Could you check a few things on this model? Use its own coordinates, in mm. A direction names the side the tool comes from. Coordinates: 2 decimals unless noted, no trailing zeros. Loops run counter-clockwise (first coordinate to the right, second up) from the corner with the lowest first, then second, coordinate; pieces in that order, holes last.
1) Imagine slicing it at A-A on x = 0. Please give me the cut outline in (y, z).
2) Imagine slicing it at B-B on z = 0. Please give me the cut outline in (x, y).
3) Imagine slicing it at C-C on y = 11.75. Please give me the cut outline in (x, z).
4) For faces 1 (the face through (3.233, 9.951, -1.341)), 2 (the face through (0, 3, 6.25)), 3 (the face through (0, 16.5, 2)), which set-ups out of +Z, -Z, +X, -X, +Y, -Y let a thin tool reach every point of the face, with its end or its side?
5) Will these pins go through, and if not, where does the flat tip stop? P1, Ø4, axis at x = -1, y = 21, coming from the +Z side; P2, Ø4, axis at y = 20.5, z = 0, coming from the +X side; P3, Ø1.5, axis at y = 22.5, z = 3, coming from the +X side; P4, Ø2, axis at x = -1, y = 11.5, coming from the +Z side.
6) Imagine slicing it at D-D on x = 2.25. Please give me the cut outline in (y, z).
7) If I drill on line 1 along X through (y, z) = (24.25, 0); line 2 along Y through (x, z) = (5.5, 2.5); line 3 along Y through (x, z) = (-1.75, -3), over which ranges is the centre line in solid material (lowest first)?
Autodesk Inventor part; units mm, degrees
ref_plane "YZ Plane" through (0, 0, 0) normal (1, 0, 0) x (0, 1, 0)
ref_plane "XZ Plane" through (0, 0, 0) normal (0, 1, 0) x (-1, 0, 0)
ref_plane "XY Plane" through (0, 0, 0) normal (0, 0, 1) x (1, 0, 0)
sketch "Sketch1" plane through (0, 0, 0) normal (0, 1, 0) x (-1, 0, 0)
  line L0 (-6.7, 6.25) -> (6.7, 6.25)
  line L1 (6.7, 6.25) -> (6.7, -6.25)
  line L2 (6.7, -6.25) -> (-6.7, -6.25)
  line L3 (-6.7, -6.25) -> (-6.7, 6.25)
  line L4 (-6.7, 6.25) -> (6.7, -6.25) construction
  line L5 (6.7, 6.25) -> (-6.7, -6.25) construction
  point P0 (0, 0)
  dimension "d0" = 13.4
  dimension "d1" = 12.5
extrude "Extrusion1" add sketch "Sketch1" along normal blind 6.5
sketch "Sketch2" plane through (0, 6.5, 0) normal (0, 1, 0) x (1, 0, 0)
  circle A0 centre (0, 0) radius 3.5
  dimension "d4" = 7
extrude "Extrusion2" add sketch "Sketch2" along normal blind 7
sketch "Sketch3" plane through (0, 13.5, 0) normal (0, 1, 0) x (1, 0, 0)
  circle A0 centre (0, 0) radius 3
  dimension "d7" = 6
extrude "Extrusion3" add sketch "Sketch3" along normal blind 13
sketch "Sketch4" plane through (0, 26.5, 0) normal (0, 1, 0) x (1, 0, 0)
  line L0 (0, -1.5) -> (2.5981, -1.5)
  circle A0 centre (0, 0) radius 3
  line L1 (0, -1.5) -> (-2.5981, -1.5)
  arc A1 (-2.5981, -1.5) -> (2.5981, -1.5) centre (0, 0) ccw
  dimension "d10" = 1.5
extrude "Extrusion4" cut sketch "Sketch4" against normal blind 10 contours L0 A0 L1 picked at (-1.5934, -1.6862)
thread "Thread1"
properties part number "PEC11R-4215F-S0024"
Filled in:
1. outline: (0, -6.25) - (6.5, -6.25) - (6.5, -3.5) - (13.5, -3.5) - (13.5, -3) - (26.5, -3) - (26.5, 1.5) - (16.5, 1.5) - (16.5, 3) - (13.5, 3) - (13.5, 3.5) - (6.5, 3.5) - (6.5, 6.25) - (0, 6.25) - close
2. outline: (-6.7, 0) - (6.7, 0) - (6.7, 6.5) - (3.5, 6.5) - (3.5, 13.5) - (3, 13.5) - (3, 26.5) - (-3, 26.5) - (-3, 13.5) - (-3.5, 13.5) - (-3.5, 6.5) - (-6.7, 6.5) - close
3. outline: circle Ø7 at (0, 0)
4. face 1: +Y
4. face 2: +Z, +X, -X, +Y, -Y
4. face 3: +Z, +X, -X, +Y
5. P1: stops at z = 1.5
5. P2: stops at x = 3
5. P3: passes through
5. P4: stops at z = 3.5
6. outline: (0, -6.25) - (6.5, -6.25) - (6.5, -2.68) - (13.5, -2.68) - (13.5, -1.98) - (26.5, -1.98) - (26.5, 1.5) - (16.5, 1.5) - (16.5, 1.98) - (13.5, 1.98) - (13.5, 2.68) - (6.5, 2.68) - (6.5, 6.25) - (0, 6.25) - close
7. line 1: x = -3 to 3
7. line 2: y = 0 to 6.5
7. line 3: y = 0 to 13.5
